Input: part model. Units: mm. Frame: model coordinates. Round coordinates to 2 decimals unless told otherwise and drop trailing zeros. Loops run counter-clockwise (first coordinate to the right, second up) from the corner with the lowest first, then second, coordinate; pieces in that order, holes last. Notation, with made-up numbers: (44, 52) -> (90, 52) arc R17 ccw to (90, 66) -> close; hole circle Ø6 at (60.5, -31.75). An arc over 180 degrees is marked (long way). Answer as a JSON object with one key per item and string values. Group by question number.
Item 1: Section query C-C on z = -1.75. Return loops of the section in (x, y).
Item 2: Pin query (flat end, axial travel): pin 1 (2 mm diameter, centred on x = 21.5, z = -1.5, fed in from +Y); pin 2 (1.2 mm diameter, centred on y = -19, z = -1.5, fed in from +X); pin 3 (2 mm diameter, centred on y = -18.5, z = -1.5, fed in from -X). Return the tip coordinate at first contact, or that it passes through.
Item 3: Material intervals for line 1 (Y direction, x = -9.5, z = -2.95); line 2 (X direction, y = 34.5, z = -2.2), sorted ascending. Write a range as [from, to].
Item 4: Section query A-A on x = 35.5. Return loops of the section in (y, z), and give its area (3 significant figures).
Item 5: Section query B-B on y = -9. Return loops of the section in (x, z), and give its area (3 significant figures).
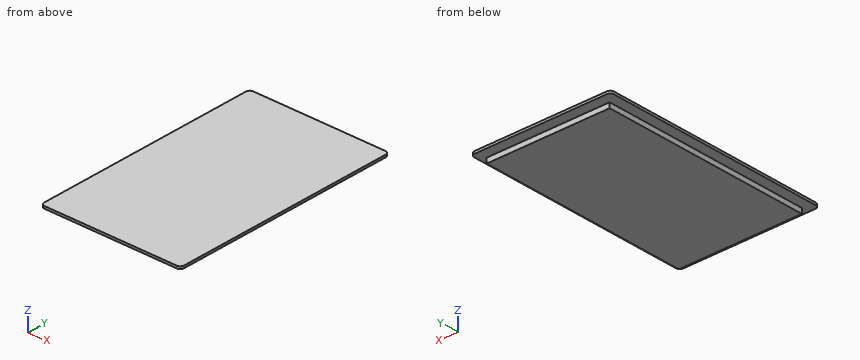
from build123d import *

# Parameters (mm, degrees)
BOSS_EXTRUDE1_DEPTH = 1.85
SKETCH2_W           = 95
SKETCH2_H           = 164
BOSS_EXTRUDE2_DEPTH = 5.75


with BuildPart() as part:
    # Sketch1 → Boss-Extrude1 (new body)
    with BuildSketch(Plane.XY):
        with BuildLine():
            Line((-51, 89), (51, 89))
            ThreePointArc((51, 89), (53.121320344, 88.121320344), (54, 86))
            Line((54, 86), (54, -86))
            ThreePointArc((54, -86), (53.121320344, -88.121320344), (51, -89))
            Line((51, -89), (-51, -89))
            ThreePointArc((-51, -89), (-53.121320344, -88.121320344), (-54, -86))
            Line((-54, -86), (-54, 86))
            ThreePointArc((-54, 86), (-53.121320344, 88.121320344), (-51, 89))
        make_face()
    extrude(amount=BOSS_EXTRUDE1_DEPTH)

    # Sketch2 → Boss-Extrude2 (add)
    with BuildSketch(Plane.XY.offset(1.85)):
        with Locations((1.5, -1)):
            Rectangle(SKETCH2_W, SKETCH2_H)
    extrude(amount=-BOSS_EXTRUDE2_DEPTH)


solid = part.part
Solved:
{
 "1": {"outline": "(-46, -83) -> (49, -83) -> (49, 81) -> (-46, 81) -> close"},
 "2": {"pin 1": "y = 81", "pin 2": "x = 49", "pin 3": "x = -46"},
 "3": {"line 1": "[-83, 81]", "line 2": "[-46, 49]"},
 "4": {"outline": "(-89, 0) -> (-83, 0) -> (-83, -3.9) -> (81, -3.9) -> (81, 0) -> (89, 0) -> (89, 1.85) -> (-89, 1.85) -> close", "area": "969 mm²"},
 "5": {"outline": "(-54, 0) -> (-46, 0) -> (-46, -3.9) -> (49, -3.9) -> (49, 0) -> (54, 0) -> (54, 1.85) -> (-54, 1.85) -> close", "area": "570 mm²"}
}
